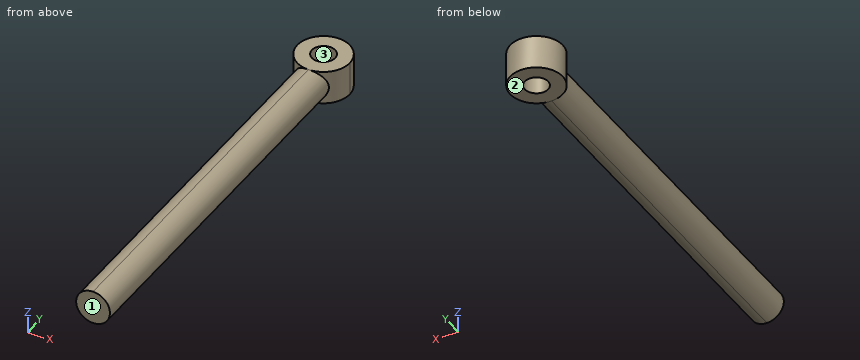
from build123d import *
from build123d.topology import SkipClean

# Parameters (mm, degrees)
SKETCH_1_R             = 5.795
EXTRUDE_1_DEPTH        = 132.19
EXTRUDE_1_2_DEPTH      = 6.19
EXTRUDE_1_2_DEPTH_BACK = 6
SKETCH_3_R             = 9
SKETCH_3_R_2           = 4
CUT_EXTRUDE_1_DEPTH    = 169.19
CUT_EXTRUDE_2_DEPTH    = 147.589618092


with BuildPart() as part:
    # 草圖1 → Extrude 1 (new body)
    with BuildSketch(Plane(origin=(0, 0, 0), x_dir=(1, 0, 0), z_dir=(0, 1, 0))):
        with Locations(Location((0, 0, 0), (0, 0, 270))):
            Circle(SKETCH_1_R)
    extrude(amount=EXTRUDE_1_DEPTH)

    # 草圖3 → Extrude 1 2 (add, two sides: drawn at the far end of the back side and taken through both)
    with BuildSketch(Plane.XY.offset(-EXTRUDE_1_2_DEPTH_BACK)):
        with Locations((0, 137.19)):
            Circle(SKETCH_3_R)
        with Locations((0, 137.19)):
            Circle(SKETCH_3_R_2, mode=Mode.SUBTRACT)
    extrude(amount=EXTRUDE_1_2_DEPTH + EXTRUDE_1_2_DEPTH_BACK)

    # 草圖7 → 除料-伸長1 (cut)
    with BuildSketch(Plane.XZ):
        Polygon((0, 5.795), (-10.217691175, 5.795), (-10.217691175, 6.299881628), (9.331279514, 6.299881628), (9.331279514, 5.795), align=None)
    extrude(amount=-CUT_EXTRUDE_1_DEPTH, mode=Mode.SUBTRACT)

    # 草圖8 → 除料-伸長2 (cut, through all)
    with SkipClean():  # the faces are left unmerged after this step: merging them gives an invalid solid
        with BuildSketch(Plane.XZ):
            Polygon((0, -5.795), (-9.78646388, -5.795), (-9.78646388, -6.666737707), (9.307322442, -6.666737707), (9.307322442, -5.795), align=None)
        extrude(amount=-CUT_EXTRUDE_2_DEPTH, mode=Mode.SUBTRACT)


solid = part.part
Check sheet for the modelled part. Datum: model origin and axes. Units: mm. Face numbers are marked on the shaded views. Round coordinates to 2 decimals unless told otherwise and drop trailing zeros. Order: outer loops, then holes, each group sorted by start corner. A loop starts at its lowest first (then second) coordinate and runs counter-clockwise, first axis right, second up.
(1) Cross-section at B-B, the plane y = 46. Enter the section's corners in (x, z) (3 decimals), and give its area (3 significant figures).
(2) Draft check along Y on the marked faces 1, 2 and 3. Enter one of: pulls with the +Y half, pulls with the -Y half, needs draft (parallel to the pull), parting line crosses it, or undercut.
(3) Scan lines: probe 1 along X at (y, z) = (137.19, -0.25); probe 2 along Y at (x, z) = (0, -0.5); probe 3 along Y at (x, z) = (-1.5, 4.75). Record each from-to range of solid material in increasing order.
(4) Cross-section at A-A, the plane z = 0. Enter the section's corners in (x, y) (3 decimals).
(5) Go/stop test with flat-tipped pins: P1, Ø1.5, axis at x = -0.5, z = 3.5, coming from the +Y side; P2, Ø1, axis at x = 2.5, z = -2.5, coming from the +Y side; P3, Ø2, axis at x = -5, z = -3, coming from the +Y side; P4, Ø6, axis at y = 111, z = 0, coming from the +X side (3 decimals). Record where each tip stops, or that it passes through.
Check sheet entries:
1. outline: circle Ø11.59 at (0, 0)
1. area: 106 mm2
2. face 1: pulls with the -Y half
2. face 2: needs draft
2. face 3: undercut
3. probe 1: x = -9 to -4, 4 to 9
3. probe 2: y = 0 to 133.19, 141.19 to 146.19
3. probe 3: y = 0 to 133.48, 140.9 to 146.06
4. outline: (-5.795, 0) - (5.795, 0) - (5.795, 130.304) arc R9 ccw (long way) to (-5.795, 130.304) - close; hole circle Ø8 at (0, 137.19)
5. P1: stops at y = 146.19
5. P2: stops at y = 145.96
5. P3: stops at y = 145.25
5. P4: stops at x = 5.795
